from build123d import *

# Parameters (mm, degrees)
SKETCH_1_R      = 5.25
EXTRUDE_1_DEPTH = 13
FILLET_1_R      = 6
FILLET_2_R      = 2
FILLET_3_R      = 3
SKETCH_2_W      = 3
SKETCH_2_H      = 13
EXTRUDE_2_DEPTH = 1.6
FILLET_4_R      = 1.4
FILLET_5_R      = 1.4
CHAMFER_1_SIZE  = 0.4


with BuildPart() as part:
    # 草图1 → 凸台-拉伸1 (new body)
    with BuildSketch(Plane(origin=(0, 0, 0), x_dir=(1, 0, 0), z_dir=(0, 1, 0))):
        with BuildLine():
            Line((5.188235294, 7.354061091), (5.188235294, 43.4))
            Line((5.188235294, 43.4), (-7.6, 43.4))
            Line((-7.6, 43.4), (-7.6, 47))
            Line((-7.6, 47), (5.4, 47))
            Line((5.4, 47), (9, 47))
            Line((9, 47), (9, 0))
            ThreePointArc((9, 0), (-7.990435459, -4.14161094), (5.188235294, 7.354061091))
        make_face()
        with Locations(Location((0, 0, 0), (0, 0, 90))):
            Circle(SKETCH_1_R, mode=Mode.SUBTRACT)
    extrude(amount=EXTRUDE_1_DEPTH)

    # 圆角1
    fillet_1_edges = [part.edges().sort_by_distance(p)[0] for p in [
        (5.188235294, 6.5, -7.354061091),
    ]]
    fillet(fillet_1_edges, radius=FILLET_1_R)

    # 圆角2
    fillet_2_edges = [part.edges().sort_by_distance(p)[0] for p in [
        (5.188235294, 6.5, -43.4),
    ]]
    fillet(fillet_2_edges, radius=FILLET_2_R)

    # 圆角3
    fillet_3_edges = [part.edges().sort_by_distance(p)[0] for p in [
        (9, 6.5, -47),
    ]]
    fillet(fillet_3_edges, radius=FILLET_3_R)

    # 草图2 → 凸台-拉伸2 (add)
    with BuildSketch(Plane.XY.offset(-43.4)):
        with Locations((-4.1, 6.5)):
            Rectangle(SKETCH_2_W, SKETCH_2_H)
    extrude(amount=EXTRUDE_2_DEPTH)

    # 圆角4
    fillet_4_edges = [part.edges().sort_by_distance(p)[0] for p in [
        (-5.6, 6.5, -41.8),
        (-2.6, 6.5, -41.8),
    ]]
    fillet(fillet_4_edges, radius=FILLET_4_R)

    # 圆角5
    fillet_5_edges = [part.edges().sort_by_distance(p)[0] for p in [
        (-2.6, 6.5, -43.4),
        (-5.6, 6.5, -43.4),
    ]]
    fillet(fillet_5_edges, radius=FILLET_5_R)

    # 倒角1
    chamfer_1_edges = [part.edges().sort_by_distance(p)[0] for p in [
        (-7.6, 6.5, -43.4),
        (-7.6, 6.5, -47),
        (0, 0, 5.25),
        (0, 13, 5.25),
        (-7.6, 13, -45.2),
        (-7.164911064, 13, -43.4),
        (-6.189364692, 0, 6.533893533),
        (-6.189364692, 13, 6.533893533),
        (3.544164316, 0, -10.851775368),
        (3.544164316, 13, -10.851775368),
        (5.188235294, 0, -28.189009248),
        (5.188235294, 13, -28.189009248),
        (4.602448856, 0, -42.814213562),
        (4.602448856, 13, -42.814213562),
        (-0.8, 0, -47),
        (-0.8, 13, -47),
        (8.121320344, 0, -46.121320344),
        (8.121320344, 13, -46.121320344),
        (-4.1, 0, -41.8),
        (-4.1, 13, -41.8),
        (-3.251668523, 13, -42.016784043),
        (-4.948331477, 0, -42.016784043),
        (-3.251668523, 0, -42.016784043),
        (0.859028711, 0, -43.4),
        (0.859028711, 13, -43.4),
        (-4.948331477, 13, -42.016784043),
        (-2.218509349, 13, -43.183215957),
        (-2.218509349, 0, -43.183215957),
        (-5.981490651, 0, -43.183215957),
        (-5.981490651, 13, -43.183215957),
        (-7.164911064, 0, -43.4),
        (-7.6, 0, -45.2),
        (9, 13, -22),
        (9, 0, -22),
    ]]
    chamfer(chamfer_1_edges, length=CHAMFER_1_SIZE)


solid = part.part
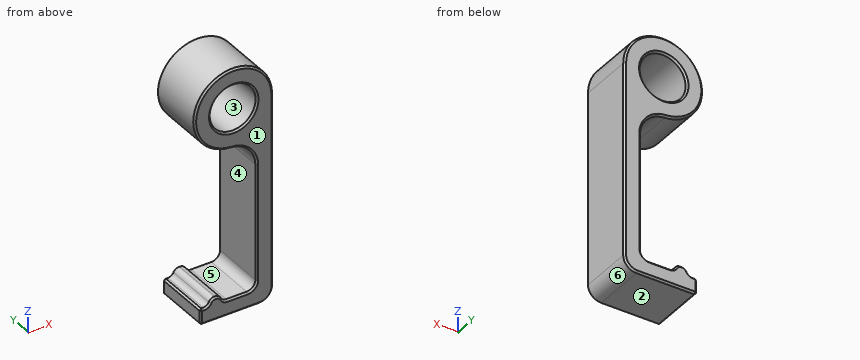
Read the model definition and answer for the solid it produces. Units are mm, in the model's axes. Face numbers are marked on the shaded views. A direction names the side the tool comes from. Coordinates: 2 decimals unless noted, no trailing zeros. Loops run counter-clockwise (first coordinate to the right, second up) from the corner with the lowest first, then second, coordinate; pieces in that order, holes last.
Q1. Consider probe 1 along X at (y, z) = (3, 0); probe 2 along Z at (x, y) = (0.5, 1); probe 3 along Z at (x, y) = (3.5, 8.75). Determine where each line is inside the solid, lowest interval first.
Q2. Which of the six approach directions +Z, -Z, +X, -X, +Y, -Y give full straight-line access (tool end or side, diameter ignored) to the marked faces 4, 5 and 6?
Q3. The part is cut by section B-B on x = 4.25. Give the number of separate pieces and of enclosed holes in the cut face, and give its area (3 significant figures).
Q4. The part is cut by section A-A on z = -30. Write down the section's boundary in (x, y), and give its area (3 significant figures).
Q5. Each of these flat-tipped pins is pushed along its axis until it touches: pin 1 Ø4 at (x, y) = (-4, 8.5) entering from +Z; pin 2 Ø1.5 at (x, y) = (5, 4.5) entering from +Z; pin 3 Ø1.4 at (y, z) = (5.5, -45) entering from -X. Where does it stop, or does it pass through?
Q6. The mould has two halves that part along Z. Classify the marked faces 1, 2 and 3: +Z half, -Z half, draft (parallel to the pull), parting line (faces both ways), or undercut.
Results below:
1. probe 1: x = -9 to -5.25, 5.25 to 9
1. probe 2: z = -47 to -43.4, -9.12 to -5.23, 5.23 to 8.99
1. probe 3: z = -47 to -43.38, -10.81 to -3.91, 3.91 to 8.29
2. face 4: -X, +Y, -Y
2. face 5: +Y, -Y
2. face 6: -Z, +X, +Y, -Y
3. separate pieces: 3
3. enclosed holes: 0
3. area: 225 mm2
4. outline: (5.19, 0.4) - (5.59, 0) - (8.6, 0) - (9, 0.4) - (9, 12.6) - (8.6, 13) - (5.59, 13) - (5.19, 12.6) - close
4. area: 49.2 mm2
5. pin 1: stops at z = 8.77
5. pin 2: stops at z = 7.93
5. pin 3: stops at x = -7.6
6. face 1: draft
6. face 2: -Z half
6. face 3: undercut
